```python
from build123d import *

# Parameters (mm, degrees)
SKETCH_W        = 82.25
SKETCH_H        = 82.25
PAD_DEPTH       = 11
PAD001_DEPTH    = 1.8
POCKET_DEPTH    = 6.5
SKETCH003_W     = 18
SKETCH003_H     = 18
SKETCH003_W_2   = 9
SKETCH003_H_2   = 9
POCKET001_DEPTH = 5
SKETCH004_R     = 2
POCKET002_DEPTH = 13
POCKET003_DEPTH = 2
SKETCH006_W     = 16.3
SKETCH006_H     = 16.3
POCKET004_DEPTH = 5


with BuildPart() as body:
    # Sketch → Pad (new body)
    with BuildSketch(Plane.XY):
        with Locations((-41.125, 41.125)):
            Rectangle(SKETCH_W, SKETCH_H)
    pad = extrude(amount=PAD_DEPTH)

    # Sketch001 (on Face5 of Pad) → Pad001 (join)
    with BuildSketch(Plane(origin=(0, 0, 0), x_dir=(1, 0, 0), z_dir=(0, 0, -1))):
        Polygon((-82.25, 0), (-82.25, -82.25), (0, -82.25), (0, -81.05), (-81.05, -81.05), (-81.05, 0), align=None)
    pad001 = extrude(amount=PAD001_DEPTH)

    # Sketch002 (on Face6 of Pad001) → Pocket (cut)
    with BuildSketch(Plane(origin=(0, 0, 11), x_dir=(0, -1, 0), z_dir=(0, 0, 1))):
        Polygon((-79.584, 0), (-79.584, -60.25), (-60.25, -60.25), (-60.25, -79.584), (0, -79.584), (0, -57.584), (-57.584, -57.584), (-57.584, 0), align=None)
    pocket = extrude(amount=-POCKET_DEPTH, mode=Mode.SUBTRACT)

    # Sketch003 (on Face7 of Pocket) → Pocket001 (cut)
    with BuildSketch(Plane.XY.offset(4.5)):
        with Locations((-45.72, 68.584)):
            Rectangle(SKETCH003_W, SKETCH003_H)
        with Locations((-22.86, 68.584)):
            Rectangle(SKETCH003_W, SKETCH003_H)
        with Locations((-4.5, 68.584)):
            Rectangle(SKETCH003_W_2, SKETCH003_H)
        with Locations((-68.584, 4.5)):
            Rectangle(SKETCH003_W, SKETCH003_H_2)
        with Locations((-68.584, 22.86)):
            Rectangle(SKETCH003_W, SKETCH003_H)
        with Locations((-68.584, 45.72)):
            Rectangle(SKETCH003_W, SKETCH003_H)
    pocket001 = extrude(amount=-POCKET001_DEPTH, mode=Mode.SUBTRACT)

    # Sketch004 (on Face2 of Pocket001) → Pocket002 (cut)
    with BuildSketch(Plane(origin=(0, 0, 0), x_dir=(1, 0, 0), z_dir=(0, 0, -1))):
        with Locations((-68.584, -68.584)):
            Circle(SKETCH004_R)
    pocket002 = extrude(amount=-POCKET002_DEPTH, mode=Mode.SUBTRACT)

    # Sketch005 (on Face2 of Pocket002) → Pocket003 (cut)
    with BuildSketch(Plane(origin=(0, 0, 0), x_dir=(1, 0, 0), z_dir=(0, 0, -1))):
        Polygon((-57.74, 0), (-57.74, -57.74), (0, -57.74), (0, -43.74), (-43.74, -43.74), (-43.74, 0), align=None)
    pocket003 = extrude(amount=-POCKET003_DEPTH, mode=Mode.SUBTRACT)

    # Sketch006 (on Face2 of Pocket003) → Pocket004 (cut)
    with BuildSketch(Plane(origin=(0, 0, 0), x_dir=(1, 0, 0), z_dir=(0, 0, -1))):
        with Locations((-8.15, -8.15)):
            Rectangle(SKETCH006_W, SKETCH006_H)
    pocket004 = extrude(amount=-POCKET004_DEPTH, mode=Mode.SUBTRACT)

    # Mirrored: Pad, Pad001, Pocket, Pocket001, Pocket002, Pocket003, Pocket004 across YZ
    add(pad.mirror(Plane.YZ))
    add(pad001.mirror(Plane.YZ))
    add(pocket.mirror(Plane.YZ), mode=Mode.SUBTRACT)
    add(pocket001.mirror(Plane.YZ), mode=Mode.SUBTRACT)
    add(pocket002.mirror(Plane.YZ), mode=Mode.SUBTRACT)
    add(pocket003.mirror(Plane.YZ), mode=Mode.SUBTRACT)
    add(pocket004.mirror(Plane.YZ), mode=Mode.SUBTRACT)


with BuildPart() as part_mirroring:
    # Part__Mirroring: instance of Body
    add(body.part.mirror(Plane(origin=(0, 0, 0), x_dir=(1, 0, 0), z_dir=(0, 1, 0))))


solid = part_mirroring.part
```
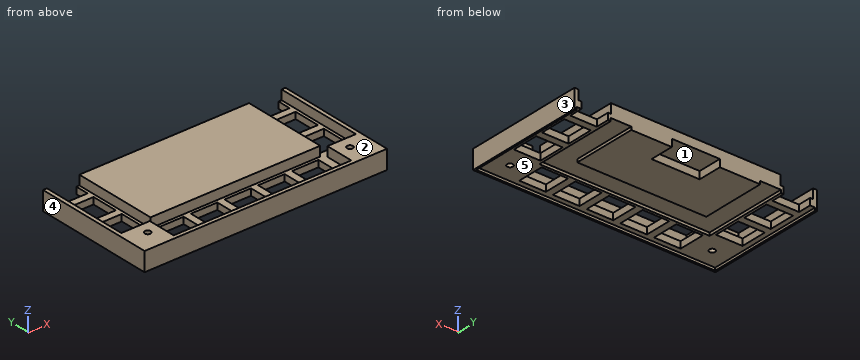
Part model, mm, in its own coordinate system. Face numbers are marked on the shaded views. A direction names the side the tool comes from. Round coordinates to 2 decimals unless told otherwise and drop trailing zeros. Loops run counter-clockwise (first coordinate to the right, second up) from the corner with the lowest first, then second, coordinate; pieces in that order, holes last.
1. Slice it at C-C (y = -23). Count the separate pieces of the cut face and the enclosed holes in it, and give its area (3 significant figures).
Solutions:
separate pieces: 3
enclosed holes: 0
area: 1,310 mm2
2. Slice it at A-A (x = -52). Give the cut face in (y, z).
Solutions:
outline: (-82.25, -1.8) - (-81.05, -1.8) - (-81.05, 0) - (-77.58, 0) - (-77.58, 4.5) - (-79.58, 4.5) - (-79.58, 11) - (-82.25, 11) - close; (-59.58, 0) - (-57.74, 0) - (-57.74, 2) - (0, 2) - (0, 11) - (-57.58, 11) - (-57.58, 4.5) - (-59.58, 4.5) - close
3. Drill centre lines: line 1 along X through (y, z) = (-23, 8.75); line 2 along X through (y, z) = (-27, 3.25); line 3 along Y through (x, z) = (-71.5, 1.5). Where is each one in solid material? Low to high.
Solutions:
line 1: x = -82.25 to -79.58, -57.58 to 57.58, 79.58 to 82.25
line 2: x = -82.25 to -77.58, -59.58 to 59.58, 77.58 to 82.25
line 3: y = -82.25 to -54.72, -36.72 to -31.86, -13.86 to -9
4. 3-axis set-ups, long thin cutter, end or side, ignore diameter. For the marked faces 4 and 5: which of +Z, -Z, +X, -X, +Y, -Y reach the whole face in a straight line?
Solutions:
face 4: +Z, -Z, -X, +Y, -Y
face 5: -Z, +Y
5. Two-plate mould, pull along X, no slides. Class the marked faces 1, 2 and 3: pulls with the +X half, pulls with the -X half, needs draft (parallel to the pull), parting line crosses it, or undercut.
Solutions:
face 1: undercut
face 2: needs draft
face 3: pulls with the +X half
6. Slice it at B-B (z = 7.5). Give the cut face in (x, y), and give its area (3 significant figures).
Solutions:
outline: (-82.25, -82.25) - (82.25, -82.25) - (82.25, 0) - (79.58, 0) - (79.58, -60.25) - (60.25, -60.25) - (60.25, -79.58) - (-60.25, -79.58) - (-60.25, -60.25) - (-79.58, -60.25) - (-79.58, 0) - (-82.25, 0) - close; (-57.58, -57.58) - (57.58, -57.58) - (57.58, 0) - (-57.58, 0) - close; hole circle Ø4 at (-68.58, -68.58); hole circle Ø4 at (68.58, -68.58)
area: 8,220 mm2
7. Slice it at D-D (x = -2). Give the cut face in (y, z), and give its area (3 significant figures).
Solutions:
outline: (-82.25, -1.8) - (-81.05, -1.8) - (-81.05, 0) - (-77.58, 0) - (-77.58, 4.5) - (-79.58, 4.5) - (-79.58, 11) - (-82.25, 11) - close; (-59.58, 0) - (-57.74, 0) - (-57.74, 2) - (-43.74, 2) - (-43.74, 0) - (-16.3, 0) - (-16.3, 5) - (0, 5) - (0, 11) - (-57.58, 11) - (-57.58, 4.5) - (-59.58, 4.5) - close
area: 573 mm2
8. Flat gauge pins, fed straight in: pin 1 (4.5 mm diameter, centred on x = -68.584, y = -68.584, fed in from +Z); pin 2 (12 mm diameter, centred on x = -41, y = -60, fed in from -Z); pin 3 (2 mm diameter, centred on x = 73, z = 8, fed in from +Y); pin 4 (5 mm diameter, centred on x = 2, z = 1.5, fed in from +Y). Where does each tip first touch, or does it go through?
Solutions:
pin 1: stops at z = 11
pin 2: stops at z = 0
pin 3: stops at y = -60.25
pin 4: stops at y = -16.3
